Design review of the part built by this model. Coordinates are the model's own, in mm. Face numbers are marked on the shaded views. A direction names the side the tool comes from. Coordinates: 2 decimals unless noted, no trailing zeros. Loops run counter-clockwise (first coordinate to the right, second up) from the corner with the lowest first, then second, coordinate; pieces in that order, holes last. Notation, with made-up numbers: M 81.5,-11 L 118.5,-11 A14 cw 118.5,3 Z; hole C 23.25,2 d4. An arc over 180 degrees is marked long. One line per item, written item: value.
```python
from build123d import *

# Parameters (mm, degrees)
CUERPO_BASE_DEPTH          = 14
CROQUIS2_R                 = 1.625
AGUJEROS_DE_SUJECION_DEPTH = 14
TUERCAS_START              = -2.5
TUERCAS_DEPTH              = 22.300472684
REDONDEO_BORDES_R          = 2
SALIENTE_EXTRUIR2_DEPTH    = 5


with BuildPart() as part:
    # Croquis1 → Cuerpo Base (new body)
    with BuildSketch(Plane(origin=(0, 0, 0), x_dir=(1, 0, 0), z_dir=(0, 1, 0))):
        Polygon((-14.55, 0), (-6.05, 0), (-6.05, 10.1), (0, 10.1), (0, 12.6), (-8.55, 12.6), (-8.55, 10.6), (-8.55, 2.5), (-11.3, 2.5), (-14.55, 2.5), align=None)
        Polygon((-8.55, 10.6), (-11.3, 2.5), (-8.55, 2.5), align=None)
        Polygon((0, 12.6), (0, 10.1), (6.05, 10.1), (6.05, 0), (14.55, 0), (14.55, 2.5), (11.3, 2.5), (8.55, 2.5), (8.55, 10.6), (8.55, 12.6), align=None)
        Polygon((11.3, 2.5), (8.55, 10.6), (8.55, 2.5), align=None)
    extrude(amount=CUERPO_BASE_DEPTH)

    # Croquis2 → Agujeros de sujecion (cut)
    with BuildSketch(Plane.XY):
        with Locations((-11.5, 7)):
            Circle(CROQUIS2_R)
        with Locations(Location((11.5, 7, 0), (0, 0, 97.069714042))):
            Circle(CROQUIS2_R)
    extrude(amount=-AGUJEROS_DE_SUJECION_DEPTH, mode=Mode.SUBTRACT)

    # Croquis3 → Tuercas (cut, through all)
    with BuildSketch(Plane.XY.offset(TUERCAS_START)):
        Polygon((-14.25, 5.41228676), (-11.5, 3.824573519), (-8.75, 5.41228676), (-8.75, 8.58771324), (-11.5, 10.175426481), (-14.25, 8.58771324), align=None)
        Polygon((11.5, 3.824573519), (14.25, 5.41228676), (14.25, 8.58771324), (11.5, 10.175426481), (8.75, 8.58771324), (8.75, 5.41228676), align=None)
    extrude(amount=-TUERCAS_DEPTH, mode=Mode.SUBTRACT)

    # Redondeo bordes
    redondeo_bordes_edges = [part.edges().sort_by_distance(p)[0] for p in [
        (-8.55, 7, -12.6),
        (8.55, 7, -12.6),
        (14.55, 0, -1.25),
        (14.55, 14, -1.25),
        (-14.55, 0, -1.25),
        (-14.55, 14, -1.25),
    ]]
    fillet(redondeo_bordes_edges, radius=REDONDEO_BORDES_R - 0.0001)  # a hair under: the kernel refuses the full size

    # Croquis4 → Saliente-Extruir2 (add)
    with BuildSketch(Plane(origin=(0, 14, 0), x_dir=(1, 0, 0), z_dir=(0, 1, 0))):
        with BuildLine():
            Line((-3.33166625, 10.1), (-6.05, 10.1))
            Line((-6.05, 10.1), (-6.05, 5.05))
            ThreePointArc((-6.05, 5.05), (-5.327245105, 7.917570329), (-3.33166625, 10.1))
        make_face()
        with BuildLine():
            Line((6.05, 10.1), (3.33166625, 10.1))
            ThreePointArc((3.33166625, 10.1), (5.327245105, 7.917570329), (6.05, 5.05))
            Line((6.05, 5.05), (6.05, 10.1))
        make_face()
    extrude(amount=-SALIENTE_EXTRUIR2_DEPTH)


solid = part.part
```
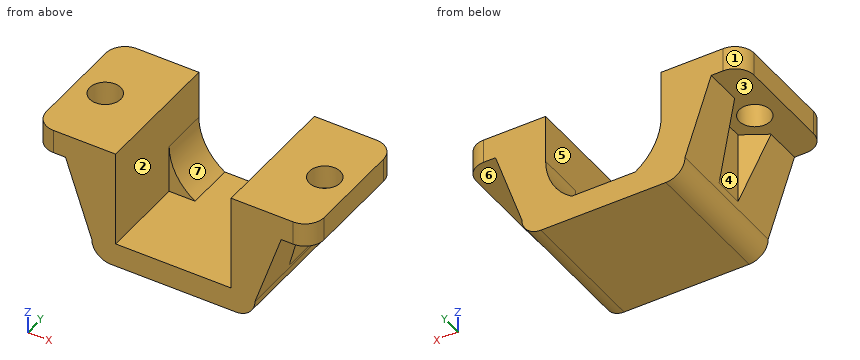
(1) We need section B-B on z = -8.5. State the section outline as (x, y) points.
Reply:
outline: M -9.26,0 L -6.05,0 L -6.05,9 L -4.97,9 L -4.97,14 L -9.26,14 L -9.26,8.88 L -8.75,8.59 L -8.75,5.41 L -9.26,5.12 Z; M 4.97,9 L 6.05,9 L 6.05,0 L 9.26,0 L 9.26,5.12 L 8.75,5.41 L 8.75,8.59 L 9.26,8.88 L 9.26,14 L 4.97,14 Z
(2) We need section C-C on y = 7. State how many separate pieces and enclosed holes the cut face has, then the cut area to 3 significant figures.
Reply:
separate pieces: 3
enclosed holes: 0
area: 108 mm2
(3) Insertion check: pin 1 (3.5 mm diameter, centred on y = 7.5, z = -8, fed in from -X); pin 2 (3.5 mm diameter, centred on y = 7.5, z = -6.5, fed in from +X); pin 3 (4.5 mm diameter, centred on x = 12.5, y = 6, fed in from -Z). Each pin has a flat end and moves straight along its axis. Give the tip position at first contact, or say it passes through.
Reply:
pin 1: stops at x = -9.66
pin 2: stops at x = 9.9
pin 3: stops at z = -2.5
(4) We need section A-A on x = -11. State the section outline as (y, z) points.
Reply:
outline: M 0,-3.38 L 4.11,-3.38 L 4.11,-2.5 L 5.45,-2.5 L 5.45,0 L 0,0 Z; M 8.55,-2.5 L 9.89,-2.5 L 9.89,-3.38 L 14,-3.38 L 14,0 L 8.55,0 Z
(5) To check wall thickness, follow line 1 along X through (y, z) = (9.75, -0.75); line 2 along Y through (x, z) = (-11.5, -1.2) (3 decimals); line 3 along Z through (x, y) = (-12.5, 4.25). State the ranges of each line that lie inside material, in increasing order. Write a range as [from, to].
Reply:
line 1: x = [-14.55, -6.05], [6.05, 14.55]
line 2: y = [0, 5.375], [8.625, 14]
line 3: z = [-2.5, 0]
(6) Tool access review of the marked faces 4, 5, 6 and 7: name each direction out of +Z, -Z, +X, -X, +Y, -Y from which nothing blocks a thin tool from reaching the whole face with its end or side.
Reply:
face 4: -Z, -X
face 5: +Z, -Y
face 6: -Z, +X
face 7: +Z, +Y, -Y
(7) We need section D-D on x = -2. State the section outline as (y, z) points, then the cut area to 3 significant figures.
Reply:
outline: M 0,-12.6 L 14,-12.6 L 14,-10.1 L 0,-10.1 Z
area: 35.0 mm2
(8) Mouldability with a two-part tool opening along X and no side actions: class the marked faces 1, 2 and 3 as released by +X, released by -X, zero draft, split by the parting line, or undercut.
Reply:
face 1: released by -X
face 2: undercut
face 3: zero draft
